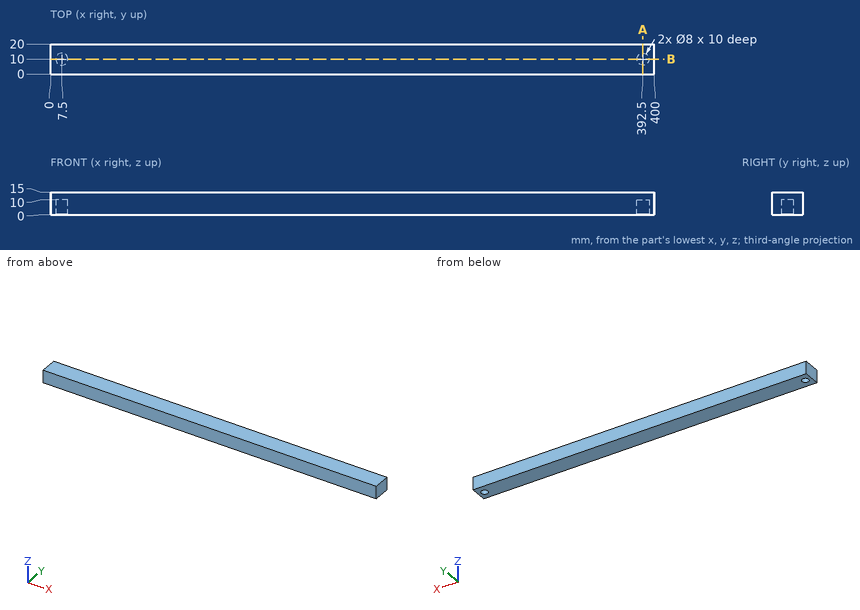
Design review of the part shown in the three views and the two pictorial views. Dimensions are in mm from the part's minimum x, y and z. Round coordinates to 2 decimals unless told otherwise and drop trailing zeros. Order: outer loops, then holes, each group sorted by start corner. A loop starts at its lowest first (then second) coordinate and runs counter-clockwise, first axis right, second up. Notation, with made-up numbers: (32.25, 62) - (45.25, 62) arc R34 ccw to (45.25, 99) - close; hole circle Ø4 at (76, 79). An arc over 180 degrees is marked (long way). Answer in a Markdown table with one row per item.
(1) Clearance check with flat-ended pins moving along their axes: P1, Ø6.5, axis at x = 392.5, y = 10, coming from the -Z side; P2, Ø5, axis at x = 128, y = 7, coming from the -Z side. State where each tip first meets the part, or that it passes through.
Result set:
| item | result |
|---|---|
| P1 | stops at z = 10 |
| P2 | stops at z = 0 |
(2) Take a section at B-B on y = 10. Write out the cut boundary in (x, z), plus the area to 3 significant figures.
Result set:
| item | result |
|---|---|
| outline | (0, 0) - (3.5, 0) - (3.5, 10) - (11.5, 10) - (11.5, 0) - (388.5, 0) - (388.5, 10) - (396.5, 10) - (396.5, 0) - (400, 0) - (400, 15) - (0, 15) - close |
| area | 5,840 mm2 |
(3) Take a section at A-A on x = 392.5. Write out the cut boundary in (y, z).
Result set:
| item | result |
|---|---|
| outline | (0, 0) - (6, 0) - (6, 10) - (14, 10) - (14, 0) - (20, 0) - (20, 15) - (0, 15) - close |
(4) For line 1 (X direction, y = 10.75, z = 3.75); line 2 (Y direction, x = 7.5, z = 7.25); line 3 (X direction, y = 13, z = 7), list the stretches that pass through material, from the lowest coordinate up. Write a range as from..to.
Result set:
| item | result |
|---|---|
| line 1 | x = 0..3.57, 11.43..388.57, 396.43..400 |
| line 2 | y = 0..6, 14..20 |
| line 3 | x = 0..4.85, 10.15..389.85, 395.15..400 |
